Verification items for the finished model (mm, model axes). A direction names the side the tool comes from. Round coordinates to 2 decimals unless told otherwise and drop trailing zeros. Order: outer loops, then holes, each group sorted by start corner. A loop starts at its lowest first (then second) coordinate and runs counter-clockwise, first axis right, second up. Notation, with made-up numbers: (61, 54.25) -> (89, 54.25) arc R24 ccw to (89, 67.25) -> close; hole circle Ø6 at (68, -11). An arc over 180 degrees is marked (long way). Return JSON: item names as keys, results as strings. Group by question number.
Item 1: Depth check by flat-ended pin: pin 1 Ø2 at (x, z) = (62.5, -14) entering from +Y; pin 2 Ø1 at (y, z) = (14, -32) entering from +X; pin 3 Ø10 at (x, y) = (38, 12.5) entering from +Z. Enter the tip coordinate at first touch or a pass-through.
Item 2: Sectioned sample at A-A on y = 15.5. Record the cut outline in (x, z), plus the area to 3 significant figures.
Item 3: Sectioned sample at C-C on x = 43.5. Record the cut outline in (y, z) (3 decimals), plus the area to 3 significant figures.
Item 4: Scan lines: probe 1 along X at (y, z) = (13.75, -31); probe 2 along Y at (x, z) = (70.5, -3); probe 3 along X at (y, z) = (5.5, -10). Record each from-to range of solid material in increasing order. Write a range as from..to.
Item 5: Sectioned sample at D-D on x = 64.5. Record the cut outline in (y, z).
Item 6: Access from +Z, -Z, +X, -X, +Y, -Y to the whole of each face (thin tool, end or side, straight path). Record for faces 4 (the cylindrical face through (41.974, 12.395, -12.477)), 5 (the flat face through (70, 10, -27)), 6 (the flat face through (45.07, 12.6, -18.8)), 7 (the flat face through (56.14, 12.6, -15.23)).
Item 7: Sectioned sample at B-B on z = -32.5. Record the cut outline in (x, y), plus the area to 3 significant figures.
Item 8: Draft check along X on faces 1 (the flat face through (19, 8, 0)), 2 (the flat face through (0, 10, -20)), 3 (the flat face through (50, 13, -30)). Enter one of: pulls with the +X half, pulls with the -X half, needs draft (parallel to the pull), parting line crosses it, or undercut.
```python
from build123d import *

# Parameters (mm, degrees)
SKETCH1_W           = 70
SKETCH1_H           = 40
BOSS_EXTRUDE1_DEPTH = 20
CUT_EXTRUDE1_DEPTH  = 15
SKETCH3_W           = 20
SKETCH3_H           = 15
CUT_EXTRUDE2_DEPTH  = 15
CUT_EXTRUDE3_DEPTH  = 15
CHAMFER1_SIZE       = 2
CHAMFER1_SIZE2      = 0.943123045
FILLET1_R           = 3
BOSS_EXTRUDE2_DEPTH = 5


with BuildPart() as part:
    # Sketch1 → Boss-Extrude1 (new body)
    with BuildSketch(Plane(origin=(0, 0, 0), x_dir=(1, 0, 0), z_dir=(0, 1, 0))):
        with Locations((35, 20)):
            Rectangle(SKETCH1_W, SKETCH1_H)
    extrude(amount=BOSS_EXTRUDE1_DEPTH)

    # Sketch2 → Cut-Extrude1 (cut)
    with BuildSketch(Plane(origin=(0, 20, 0), x_dir=(1, 0, 0), z_dir=(0, 1, 0))):
        Polygon((20, 15), (20, 37.5), (50, 37.5), (50, 22.5), (40, 15), align=None)
    extrude(amount=-CUT_EXTRUDE1_DEPTH, mode=Mode.SUBTRACT)

    # Sketch3 → Cut-Extrude2 (cut)
    with BuildSketch(Plane(origin=(0, 20, 0), x_dir=(1, 0, 0), z_dir=(0, 1, 0))):
        with Locations((30, 7.5)):
            Rectangle(SKETCH3_W, SKETCH3_H)
    extrude(amount=-CUT_EXTRUDE2_DEPTH, mode=Mode.SUBTRACT)

    # Sketch4 → Cut-Extrude3 (cut)
    with BuildSketch(Plane(origin=(0, 20, 0), x_dir=(1, 0, 0), z_dir=(0, 1, 0))):
        Polygon((40, 12), (70, 18), (70, 0), (40, 0), align=None)
    extrude(amount=-CUT_EXTRUDE3_DEPTH, mode=Mode.SUBTRACT)

    # Chamfer1
    chamfer1_edges = [part.edges().sort_by_distance(p)[0] for p in [
        (40, 12.5, -12),
    ]]
    chamfer1_side = [part.faces().sort_by_distance(p)[0] for p in [
        (55, 12.5, -15),
    ]]
    chamfer(chamfer1_edges, length=CHAMFER1_SIZE, length2=CHAMFER1_SIZE2, reference=chamfer1_side[0])

    # Fillet1
    fillet1_edges = [part.edges().sort_by_distance(p)[0] for p in [
        (41.961161351, 12.5, -12.39223227),
    ]]
    fillet(fillet1_edges, radius=FILLET1_R)

    # Sketch5 → Boss-Extrude2 (add)
    with BuildSketch(Plane.XZ):
        with BuildLine():
            Line((70, -15), (70, 0))
            ThreePointArc((70, 0), (75.077747211, -7.5), (70, -15))
        make_face()
    extrude(amount=-BOSS_EXTRUDE2_DEPTH)


solid = part.part
```
Recorded:
{
 "1": {"pin 1": "y = 5", "pin 2": "x = 70", "pin 3": "z = -12.48"},
 "2": {"outline": "(0, -40) -> (70, -40) -> (70, -18) -> (42.67, -12.53) arc R3 ccw to (41.27, -12.59) -> (40, -12.94) -> (40, -15) -> (50, -22.5) -> (50, -37.5) -> (20, -37.5) -> (20, 0) -> (0, 0) -> close", "area": "1,410 mm²"},
 "3": {"outline": "(0, -40) -> (20, -40) -> (20, -37.5) -> (5, -37.5) -> (5, -17.625) -> (20, -17.625) -> (20, -12.7) -> (5, -12.7) -> (5, 0) -> (0, 0) -> close", "area": "311 mm²"},
 "4": {"probe 1": "0..20, 50..70", "probe 2": "0..5", "probe 3": "0..20"},
 "5": {"outline": "(0, -40) -> (20, -40) -> (20, -16.9) -> (5, -16.9) -> (5, 0) -> (0, 0) -> close"},
 "6": {"face 4": "+Z, +Y", "face 5": "-Z, +X, +Y, -Y", "face 6": "+Y", "face 7": "+Z, +X, +Y"},
 "7": {"outline": "(0, 0) -> (70, 0) -> (70, 20) -> (50, 20) -> (50, 5) -> (20, 5) -> (20, 20) -> (0, 20) -> close", "area": "950 mm²"},
 "8": {"face 1": "needs draft", "face 2": "pulls with the -X half", "face 3": "undercut"}
}
